Can you work these out from the drawing? Everything is in mm from the part's minimum corner. A direction names the side the tool comes from. Give positions to 0.01 mm unless a question says otherwise; leave off trailing zeros. Return JSON: item names as keys, results as strings.
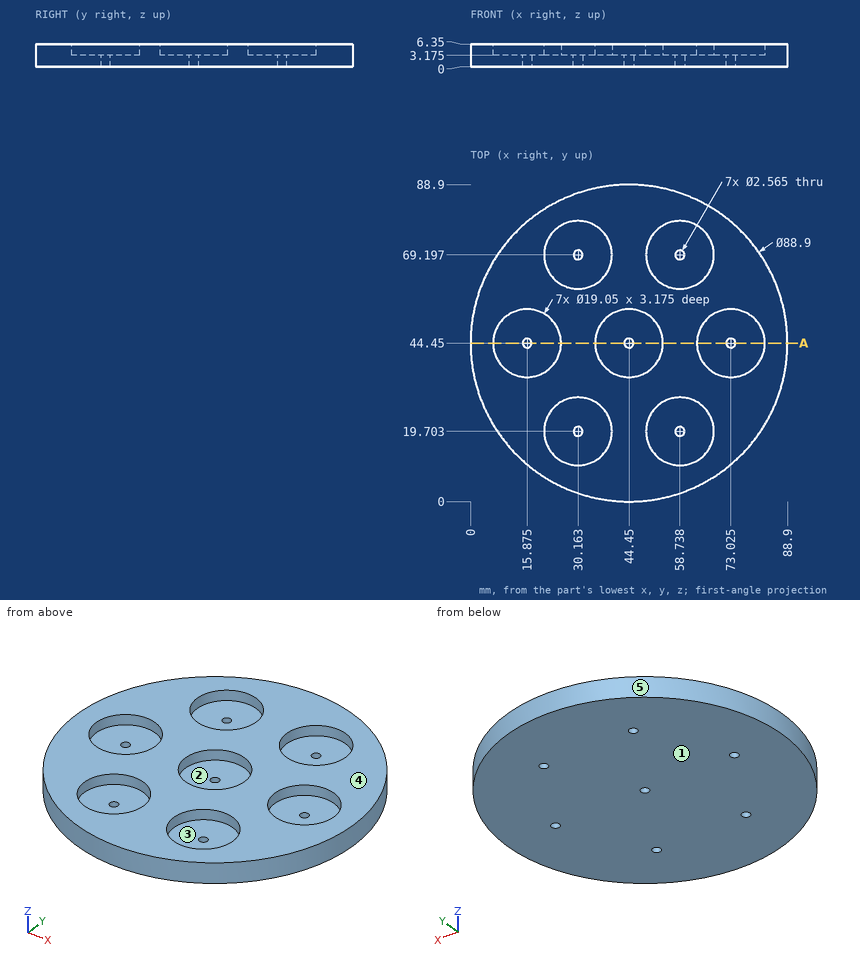
1. Suppose I cut it at A-A, the plane y = 44.45. Count the separate pieces of the cut face and the enclosed holes in it.
Taken from the geometry:
{"separate pieces": "4", "enclosed holes": "0"}
2. If we mould it in two halves opening along X, with no side actions, what happens to the marked faces 3, 4 and 5? For each: released by +X, released by -X, zero draft, split by the parting line, or undercut.
Taken from the geometry:
{"face 3": "undercut", "face 4": "zero draft", "face 5": "split by the parting line"}
3. Which directions (+Z, -Z, +X, -X, +Y, -Y) give clear straight access to the entire face, cutting with the end or side of a thin tool? Please do the marked faces 1 and 2.
Taken from the geometry:
{"face 1": "-Z, +X, -X, +Y, -Y", "face 2": "+Z"}
4. For pin 1 Ø2 at (x, y) = (15.875, 44.45) entering from +Z; pin 2 Ø2 at (x, z) = (60, 5) entering from +Y; pin 3 Ø11.5 at (x, y) = (58.74, 69.2) entering from -Z; pin 4 Ø2 at (x, z) = (50, 1.5) entering from -Y, each with a flat end and sliding along its axis, tell me the tip position at first contact or that it passes through.
Taken from the geometry:
{"pin 1": "passes through", "pin 2": "stops at y = 86.45", "pin 3": "stops at z = 0", "pin 4": "stops at y = 0.23"}
5. If I drill on line 1 (Y direction, x = 37, z = 5.5) (1 decimal); line 2 (X direction, y = 41.5, z = 5); line 3 (X direction, y = 25, z = 5.75) (1 decimal), over which ranges is the centre line in solid material (lowest first)? Write a range as [from, to].
Taken from the geometry:
{"line 1": "y = [0.6, 13.1], [26.3, 38.5], [50.4, 62.6], [75.8, 88.3]", "line 2": "x = [0.1, 6.82], [24.93, 35.39], [53.51, 63.97], [82.08, 88.8]", "line 3": "x = [4.5, 22.2], [38.1, 50.8], [66.7, 84.4]"}
